Geometry: final body of the model. Coordinates: model frame, mm. Face numbers are marked on the shaded views. Coordinates: 2 decimals unless noted, no trailing zeros. Order: outer loops, then holes, each group sorted by start corner. A loop starts at its lowest first (then second) coordinate and runs counter-clockwise, first axis right, second up. Notation, with made-up numbers: M -26.5,22.25 L 20.5,22.25 A17 cw 20.5,40.25 Z; hole C 43,44 d3. An arc over 180 degrees is marked long. One line per question, with ' | ' between items.
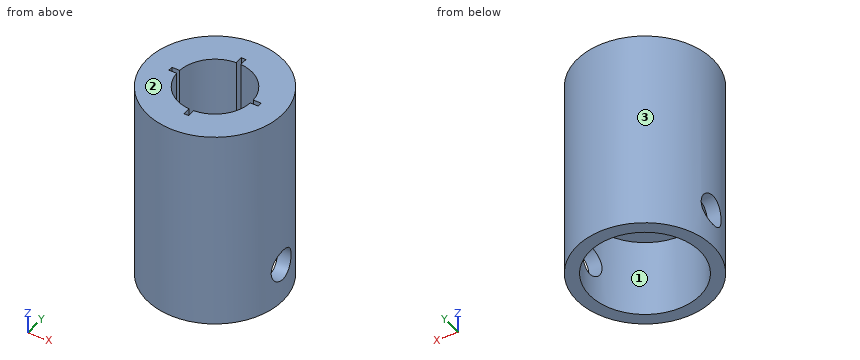
from build123d import *

# Parameters (mm, degrees)
SKETCH_1_R               = 8.75
SKETCH_1_R_2             = 7.1
EXTRUDE_1_DEPTH          = 10
CUT_EXTRUDE_1_DEPTH      = 20
CUT_EXTRUDE_1_DEPTH_BACK = 10
SKETCH_2_R               = 2
SKETCH_3_R               = 8.75
SKETCH_3_R_2             = 4.75
EXTRUDE_2_DEPTH          = 16
CUT_EXTRUDE_START        = -8
CUT_EXTRUDE_2_DEPTH      = 8


with BuildPart() as part:
    # 草图1 → 凸台-拉伸1 (new body)
    with BuildSketch(Plane.XY):
        Circle(SKETCH_1_R)
        Circle(SKETCH_1_R_2, mode=Mode.SUBTRACT)
    extrude(amount=EXTRUDE_1_DEPTH)

    # 草图2 → 切除-拉伸1 (cut, two sides: drawn at the far end of the back side and taken through both)
    with BuildSketch(Plane(origin=(0, 0, 0), x_dir=(0, 0, -1), z_dir=(1, 0, 0)).offset(-CUT_EXTRUDE_1_DEPTH_BACK)):
        with Locations((-5, 0)):
            Circle(SKETCH_2_R)
    extrude(amount=CUT_EXTRUDE_1_DEPTH + CUT_EXTRUDE_1_DEPTH_BACK, mode=Mode.SUBTRACT)

    # 草图3 → 凸台-拉伸2 (add)
    with BuildSketch(Plane.XY.offset(10)):
        Circle(SKETCH_3_R)
        Circle(SKETCH_3_R_2, mode=Mode.SUBTRACT)
    extrude(amount=EXTRUDE_2_DEPTH)

    # 草图4 → 切除-拉伸2 (cut)
    with BuildSketch(Plane.XY.offset(26).offset(CUT_EXTRUDE_START)):
        with BuildLine():
            Line((-0.3, -4.740516849), (-0.3, -5.75))
            Line((-0.3, -5.75), (0.3, -5.75))
            Line((0.3, -5.75), (0.3, -4.740516849))
            ThreePointArc((0.3, -4.740516849), (0, -4.75), (-0.3, -4.740516849))
        make_face()
        with BuildLine():
            Line((-5.75, -0.3), (-4.740516849, -0.3))
            ThreePointArc((-4.740516849, -0.3), (-4.75, 0), (-4.740516849, 0.3))
            Line((-4.740516849, 0.3), (-5.75, 0.3))
            Line((-5.75, 0.3), (-5.75, -0.3))
        make_face()
        with BuildLine():
            Line((-0.3, 5.75), (-0.3, 4.740516849))
            ThreePointArc((-0.3, 4.740516849), (0, 4.75), (0.3, 4.740516849))
            Line((0.3, 4.740516849), (0.3, 5.75))
            Line((0.3, 5.75), (-0.3, 5.75))
        make_face()
        with BuildLine():
            Line((5.75, 0.3), (4.740516849, 0.3))
            ThreePointArc((4.740516849, 0.3), (4.75, 0), (4.740516849, -0.3))
            Line((4.740516849, -0.3), (5.75, -0.3))
            Line((5.75, -0.3), (5.75, 0.3))
        make_face()
    extrude(amount=CUT_EXTRUDE_2_DEPTH, mode=Mode.SUBTRACT)


solid = part.part
1. Section B-B, the plane z = 22.75. Output: boundary loops of the cut face in (x, y), and give its area (3 significant figures).
Response values:
outline: C 0,0 d17.5; hole M -5.75,-0.3 L -4.74,-0.3 A4.75 ccw -0.3,-4.74 L -0.3,-5.75 L 0.3,-5.75 L 0.3,-4.74 A4.75 ccw 4.74,-0.3 L 5.75,-0.3 L 5.75,0.3 L 4.74,0.3 A4.75 ccw 0.3,4.74 L 0.3,5.75 L -0.3,5.75 L -0.3,4.74 A4.75 ccw -4.74,0.3 L -5.75,0.3 Z | area: 167 mm^2
2. Section C-C, the plane x = 0. Output: boundary loops of the cut face in (y, z), and give its area (3 significant figures).
Response values:
outline: M -8.75,0 L -7.1,0 L -7.1,10 L -4.75,10 L -4.75,18 L -5.75,18 L -5.75,26 L -8.75,26 Z; M 4.75,10 L 7.1,10 L 7.1,0 L 8.75,0 L 8.75,26 L 5.75,26 L 5.75,18 L 4.75,18 Z | area: 145 mm^2
3. Material intervals for line 1 (X direction, y = 0, z = 7.75); line 2 (Y direction, x = 0.25, z = 16.75), sorted ascending. Write a range as [from, to].
Response values:
line 1: x = [-8.75, -7.1], [7.1, 8.75] | line 2: y = [-8.75, -4.74], [4.74, 8.75]
4. Pin query (flat end, axial travel): P1, Ø1.1, axis at x = 5, z = 21, coming from the -Y side; P2, Ø3, axis at y = 3.5, z = 10, coming from the +X side; P3, Ø7, axis at x = -1.5, y = 1.5, coming from the -Z side; P4, Ø1, axis at x = 3.5, y = 2, coming from the +Z side. Return the tip coordinate at first contact, or that it passes through.
Response values:
P1: stops at y = -7.53 | P2: stops at x = 8.52 | P3: stops at z = 10 | P4: passes through
5. Section D-D, the plane z = 5. Output: boundary loops of the cut face in (x, y), and give its area (3 significant figures).
Response values:
outline: M -8.52,-2 A8.75 ccw 8.52,-2 L 6.81,-2 A7.1 cw -6.81,-2 Z; M -8.52,2 L -6.81,2 A7.1 cw 6.81,2 L 8.52,2 A8.75 ccw Z | area: 68.8 mm^2
6. Section A-A, the plane y = 0. Output: boundary loops of the cut face in (x, z).
Response values:
outline: M -8.75,0 L -7.1,0 L -7.1,3 L -8.75,3 Z; M -8.75,7 L -7.1,7 L -7.1,10 L -4.75,10 L -4.75,18 L -5.75,18 L -5.75,26 L -8.75,26 Z; M 4.75,10 L 7.1,10 L 7.1,7 L 8.75,7 L 8.75,26 L 5.75,26 L 5.75,18 L 4.75,18 Z; M 7.1,0 L 8.75,0 L 8.75,3 L 7.1,3 Z
7. Draft query along Y for the marked faces 1, 2 and 3. Return one class per face: pulls with the +Y half, pulls with the -Y half, needs draft (parallel to the pull), parting line crosses it, or undercut.
Response values:
face 1: undercut | face 2: needs draft | face 3: parting line crosses it
